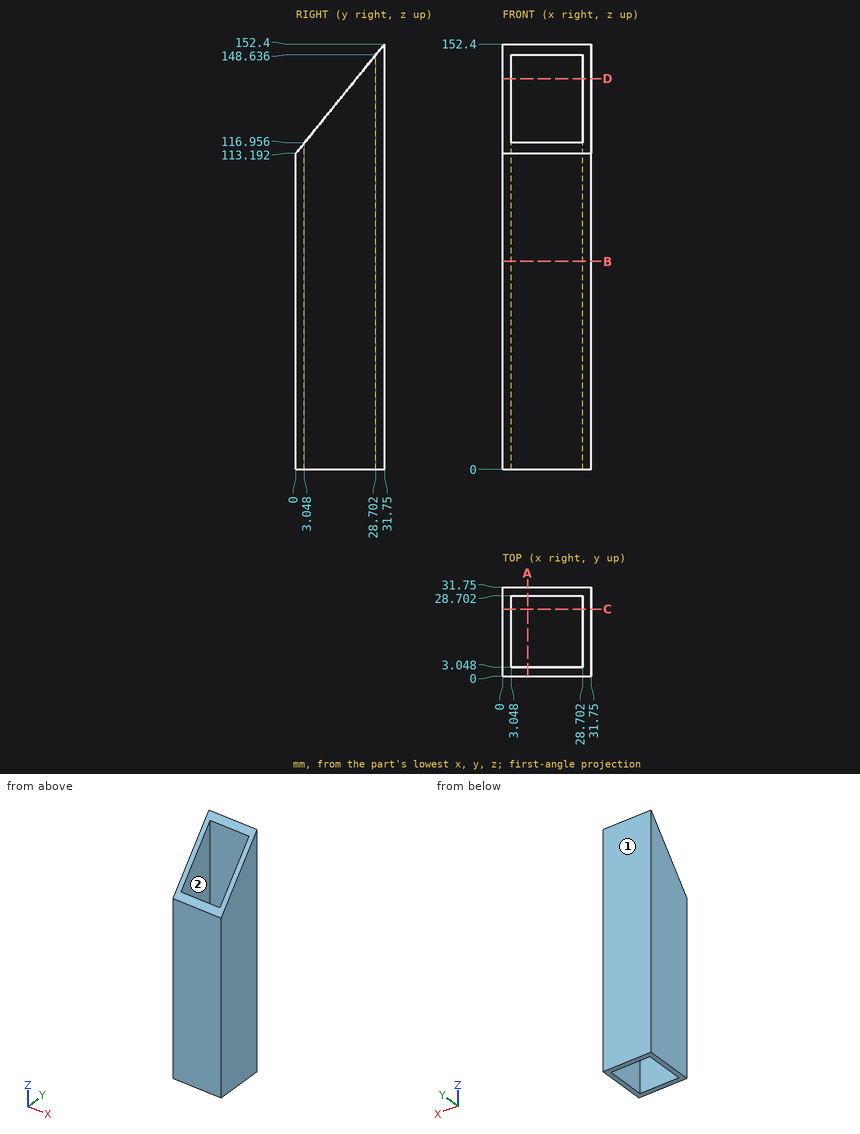
Geometry check sheet. Reference: drawing and pictorial views, mm from the part's lowest x, y, z. A direction names the side the tool comes from. Give positions to 0.01 mm unless a question says otherwise; leave off trailing zeros. Order: outer loops, then holes, each group sorted by start corner. A loop starts at its lowest first (then second) coordinate and runs counter-clockwise, first axis right, second up. Notation, with made-up numbers: (88.5, 65.5) -> (105.5, 65.5) arc R33 ccw to (105.5, 96.5) -> close; hole circle Ø2 at (87.25, -3.75). An arc over 180 degrees is marked (long way). Write each question's results on one line, items separated by ' | '. Start each with the question number.
(1) Access from +Z, -Z, +X, -X, +Y, -Y to the whole of each face (thin tool, end or side, straight path). Record for the marked faces 1 and 2.
(2) Sectioned sample at B-B (z = 74.5). Enter the section's corners in (x, y), plus the area to 3 significant figures.
(3) Sectioned sample at C-C (y = 24). Enter the section's corners in (x, z), plus the area to 3 significant figures.
(4) Gauge pin test, flat end, axial feed: P1, Ø1, axis at x = 4.5, y = 13, coming from the -Z side. Record the tip position at first contact, or that the pin passes through.
(5) Sectioned sample at A-A (x = 9). Enter the section's corners in (y, z).
(6) Sectioned sample at D-D (z = 140). Enter the section's corners in (x, y), plus the area to 3 significant figures.
(7) Scan lines: line 1 (X direction, y = 10, z = 24.5); line 2 (Y direction, x = 6, z = 141). Record each from-to range of solid material in increasing order.
Answer below:
1) face 1: +Z, -Z, +X, -X, +Y | face 2: +Z, -Z
2) outline: (0, 0) -> (31.75, 0) -> (31.75, 31.75) -> (0, 31.75) -> close; hole (3.05, 3.05) -> (28.7, 3.05) -> (28.7, 28.7) -> (3.05, 28.7) -> close | area: 350 mm2
3) outline: (0, 0) -> (3.05, 0) -> (3.05, 142.83) -> (0, 142.83) -> close; (28.7, 0) -> (31.75, 0) -> (31.75, 142.83) -> (28.7, 142.83) -> close | area: 871 mm2
4) P1: through
5) outline: (0, 0) -> (3.05, 0) -> (3.05, 116.96) -> (0, 113.19) -> close; (28.7, 0) -> (31.75, 0) -> (31.75, 152.4) -> (28.7, 148.64) -> close
6) outline: (0, 21.71) -> (3.05, 21.71) -> (3.05, 28.7) -> (28.7, 28.7) -> (28.7, 21.71) -> (31.75, 21.71) -> (31.75, 31.75) -> (0, 31.75) -> close | area: 139 mm2
7) line 1: 0 to 3.05, 28.7 to 31.75 | line 2: 28.7 to 31.75
